```python
from build123d import *

# Parameters (mm, degrees)
BOSS_EXTRUDE2_DEPTH = 10
SKETCH6_R           = 1.636760028
CUT_EXTRUDE1_DEPTH  = 27
SKETCH7_R           = 1.638016743
CUT_EXTRUDE2_DEPTH  = 27
SKETCH8_R           = 1.650737017
CUT_EXTRUDE3_DEPTH  = 27
SKETCH14_R          = 2.003260407
CUT_EXTRUDE4_DEPTH  = 27


with BuildPart() as part:
    # Sketch2 → Boss-Extrude2 (new body)
    with BuildSketch(Plane.XY.offset(16)):
        Polygon((-14.961915992, 18.349138456), (-14.957534249, -8.487840275), (284.912453053, -8.438879726), (284.90807131, 18.398099005), align=None)
    extrude(amount=BOSS_EXTRUDE2_DEPTH)

    # Sketch6 → Cut-Extrude1 (cut)
    with BuildSketch(Plane(origin=(0, 0, 16), x_dir=(-1, 0, 0), z_dir=(0, 0, -1))):
        with Locations((-135.00258755, -0.00593878)):
            Circle(SKETCH6_R)
    extrude(amount=-CUT_EXTRUDE1_DEPTH, mode=Mode.SUBTRACT)

    # Sketch7 → Cut-Extrude2 (cut)
    with BuildSketch(Plane(origin=(0, 0, 16), x_dir=(-1, 0, 0), z_dir=(0, 0, -1))):
        with Locations((-269.998815676, -0.007408264)):
            Circle(SKETCH7_R)
    extrude(amount=-CUT_EXTRUDE2_DEPTH, mode=Mode.SUBTRACT)

    # Sketch8 → Cut-Extrude3 (cut)
    with BuildSketch(Plane(origin=(0, 0, 16), x_dir=(-1, 0, 0), z_dir=(0, 0, -1))):
        with Locations((-0.005146572, -0.011071128)):
            Circle(SKETCH8_R)
    extrude(amount=-CUT_EXTRUDE3_DEPTH, mode=Mode.SUBTRACT)

    # Sketch14 → Cut-Extrude4 (cut)
    with BuildSketch(Plane(origin=(-0.00299631, 18.351580838, 0), x_dir=(0.9999999866710311, 0.00016327258684284348, 0), z_dir=(-0.00016327258684284348, 0.9999999866710311, 0))):
        with Locations(Location((-6.872916807, -21.024902159, 0), (0, 0, 180))):
            Circle(SKETCH14_R)
        with Locations(Location((57.127083193, -21.024902159, 0), (0, 0, 180))):
            Circle(SKETCH14_R)
        with Locations(Location((121.127083193, -21.024902159, 0), (0, 0, 180))):
            Circle(SKETCH14_R)
        with Locations(Location((153.127083193, -21.024902159, 0), (0, 0, 180))):
            Circle(SKETCH14_R)
        with Locations(Location((217.127083193, -21.024902159, 0), (0, 0, 180))):
            Circle(SKETCH14_R)
        with Locations(Location((281.127083193, -21.024902159, 0), (0, 0, 180))):
            Circle(SKETCH14_R)
    extrude(amount=-CUT_EXTRUDE4_DEPTH, mode=Mode.SUBTRACT)


solid = part.part
```
Verification items for the finished model (mm, model axes). Round coordinates to 2 decimals unless told otherwise and drop trailing zeros.
1. Scan lines: L1, parallel to X at y = 1, z = 17; L2, parallel to Y at x = 263.5, z = 20.25; L3, parallel to X at y = -5.75, z = 16.5. Record each from-to range of solid material in increasing order.
2. Section check A-A on y = 6. State how many separate pieces and enclosed holes the cut face has, plus the area to 3 significant figures.
3. Gauge pin test, flat ends, axial feed: P1, Ø2, axis at x = 86.5, z = 24, coming from the +Y side; P2, Ø2, axis at x = 0.01, y = -0.01, coming from the +Z side; P3, Ø4, axis at y = -5, z = 22.5, coming from the -X side; P4, Ø2, axis at x = 130, z = 20, coming from the -Y side. Record the tip position at first contact, or that the pin passes through.
Answer:
1. L1: x = -14.96 to -1.3, 1.31 to 133.71, 136.29 to 268.71, 271.29 to 284.91
1. L2: y = -8.44 to 18.39
1. L3: x = -14.96 to 284.91
2. separate pieces: 1
2. enclosed holes: 6
2. area: 2,920 mm2
3. P1: stops at y = 18.37
3. P2: passes through
3. P3: stops at x = -14.96
3. P4: stops at y = -8.46
